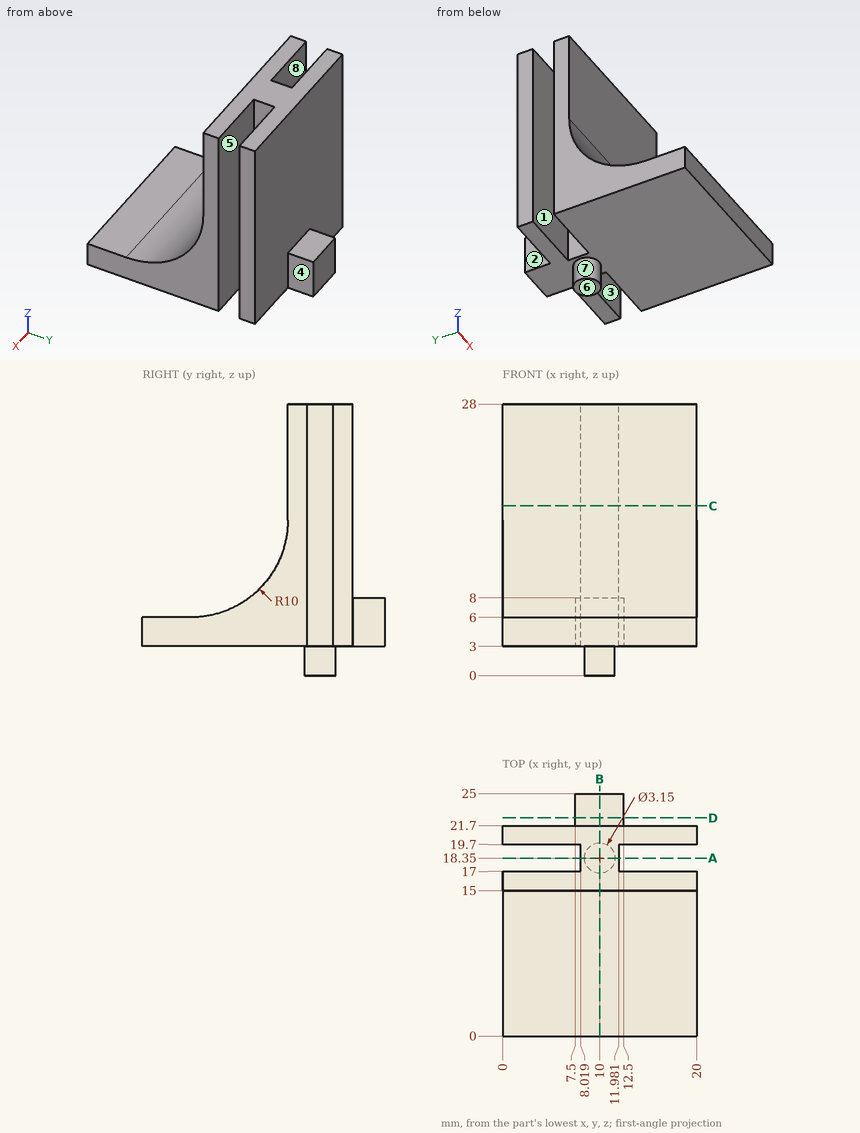
Here's the drawing with two shaded views (mm, measured from the low corner). I have some questions. A direction names the side the tool comes from. Coordinates: 2 decimals unless noted, no trailing zeros. Loops run counter-clockwise (first coordinate to the right, second up) from the corner with the lowest first, then second, coordinate; pieces in that order, holes last. Notation, with made-up numbers: (-2, -35) -> (33, -35) arc R22 ccw to (33, 0) -> close; hole circle Ø4 at (60.25, 68). An arc over 180 degrees is marked (long way). Use one line per item in the form item = value. Start each with the question number.
(1) Please list where these lines run through material, in increasing order: line 1 along Y through (x, z) = (2.5, 15.75); line 2 along Y through (x, z) = (18.5, 5.75); line 3 along Z through (x, y) = (11.25, 2.5).
(2) If we section it at B-B (x = 10): Please give me the cut outline in (y, z) (1 decimal), then the cut area to 3 significant figures.
(3) Will these pins go through, and if not, where does the flat tip stop? pin 1 (10 mm diameter, centred on x = 12, z = 21.5, fed in from +Y); pin 2 (1 mm diameter, centred on y = 23, z = 6.5, fed in from +X); pin 3 (5.5 mm diameter, centred on x = 9.5, y = 2.5, fed in from +Z); pin 4 (4 mm diameter, centred on y = 12, z = 15, fed in from -X).
(4) If we section it at D-D (y = 22.5): Please give me the cut outline in (x, z).
(5) If we section it at C-C (z = 17.5): Please give me the cut outline in (x, y).
(6) On a 3-axis mill with a long thin cutter (end or side, diameter ignored), from which of +Z, -Z, +X, -X, +Y, -Y can I reach the whole of each face in a straight line? I mean the marked faces 1, 2, 3 and 4. Say none if no direction works.
(7) If we section it at A-A (y = 18.35): Please give me the cut outline in (x, z) (1 decimal).
(8) We'd pull the mould along Y, two halves only. Please class the marked faces 5, 6, 7 and 8: pulls with the +Y half, pulls with the -Y half, needs draft (parallel to the pull), parting line crosses it, or undercut.
Verdict:
q1.line_1 = 15 to 17, 19.7 to 21.7
q1.line_2 = 0 to 17, 19.7 to 21.7
q1.line_3 = 3 to 6
q2.outline = (0, 3) -> (16.8, 3) -> (16.8, 0) -> (19.9, 0) -> (19.9, 3) -> (25, 3) -> (25, 8) -> (21.7, 8) -> (21.7, 28) -> (15, 28) -> (15, 16) arc R10 cw to (5, 6) -> (0, 6) -> close
q2.area = 260 mm²
q3.pin_1 = 21.7
q3.pin_2 = 12.5
q3.pin_3 = 6
q3.pin_4 = through
q4.outline = (7.5, 3) -> (12.5, 3) -> (12.5, 8) -> (7.5, 8) -> close
q5.outline = (0, 15) -> (20, 15) -> (20, 17) -> (11.98, 17) -> (11.98, 19.7) -> (20, 19.7) -> (20, 21.7) -> (0, 21.7) -> (0, 19.7) -> (8.02, 19.7) -> (8.02, 17) -> (0, 17) -> close
q6.face_1 = +Z, -Z, -X
q6.face_2 = +Z, -Z, -X, +Y
q6.face_3 = +Z, -Z, +X
q6.face_4 = +Z, -Z, +X, +Y
q7.outline = (8, 3) -> (8.4, 3) -> (8.4, 0) -> (11.6, 0) -> (11.6, 3) -> (12, 3) -> (12, 28) -> (8, 28) -> close
q8.face_5 = undercut
q8.face_6 = needs draft
q8.face_7 = parting line crosses it
q8.face_8 = undercut
